Input: dimensioned drawing with shaded views. Units: mm. Origin: part minimum x, y, z. A direction names the side the tool comes from. Coordinates: 2 decimals unless noted, no trailing zeros. Order: outer loops, then holes, each group sorted by start corner. A loop starts at its lowest first (then second) coordinate and runs counter-clockwise, first axis right, second up. Notation, with made-up numbers: (13, 13.5) - (41, 13.5) arc R27 ccw to (41, 30.5) - close; hole circle Ø10 at (-16, -26.5). An arc over 180 degrees is marked (long way). Answer as CSV lines item,"result". Start each with the question number.
Item 1: Section B-B (x = 72). Output: boundary loops of the cut face in (y, z), and give its area (3 significant figures).
Item 2: Section D-D (z = 65). Output: boundary loops of the cut face in (x, y), and give its area (4 significant figures).
Item 3: First-contact query: pin 1 (12 mm diameter, centred on x = 56, y = 11.5, fed in from -Z) (1 decimal); pin 2 (6 mm diameter, centred on x = 43, y = 82, fed in from -Z). Flat tips, straight axial feed; report the tip coordinate or a pass-through.
Item 4: Access query for the marked faces 1, 2, 3, 4 and 5. Directions: +Z, -Z, +X, -X, +Y, -Y. A direction counts if a zero-diameter tool reaches every point of the face in a straight line with its end or side. Return the directions, or none.
Item 5: Draft query along Y for the marked faces 6, 7 and 8. Return one class per face: +Y half, -Y half, draft (parallel to the pull), parting line (faces both ways), or undercut.
Item 6: Section A-A (z = 41). Output: boundary loops of the cut face in (x, y), and give its area (3 significant figures).
Item 7: Material intervals for line 1 along Y through (x, z) = (45.5, 50); line 2 along X through (y, z) = (44, 22), sorted ascending.
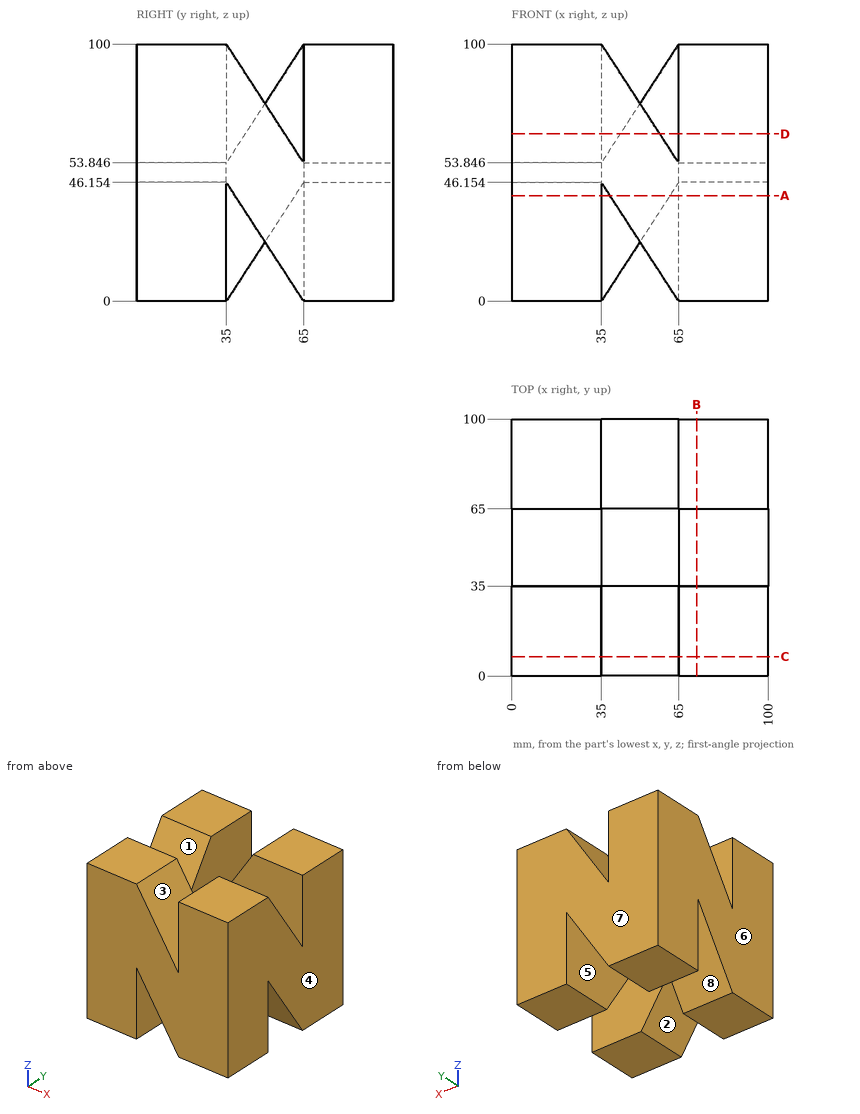
Determined:
1,outline,"(0, 0) - (35, 0) - (35, 46.15) - (65, 0) - (100, 0) - (100, 100) - (65, 100) - (65, 53.85) - (35, 100) - (0, 100) - close"
1,area,"8,620 mm^2"
2,outline,"(0, 0) - (57.75, 0) - (57.75, 35) - (0, 35) - close; (0, 42.25) - (35, 42.25) - (35, 100) - (0, 100) - close; (42.25, 65) - (100, 65) - (100, 100) - (42.25, 100) - close; (65, 0) - (100, 0) - (100, 57.75) - (65, 57.75) - close"
2,area,"8,085 mm^2"
3,pin 1,"stops at z = 4.6"
3,pin 2,"stops at z = 7.69"
4,face 1,"+Z, -X"
4,face 2,"-Z, -Y"
4,face 3,"+Z, -Y"
4,face 4,"+Z, -Z, +X, +Y, -Y"
4,face 5,"none"
5,face 6,"draft"
5,face 7,"+Y half"
5,face 8,"undercut"
6,outline,"(0, 0) - (35, 0) - (35, 61.65) - (0, 61.65) - close; (0, 65) - (61.65, 65) - (61.65, 100) - (0, 100) - close; (38.35, 0) - (100, 0) - (100, 35) - (38.35, 35) - close; (65, 38.35) - (100, 38.35) - (100, 100) - (65, 100) - close"
6,area,"8,630 mm^2"
7,line 1,"y = 0 to 35, 65 to 100"
7,line 2,"x = 0 to 35"
